from build123d import *

# Parameters (mm, degrees)
F1_DEPTH = 152.4
F2_T     = -6.35


with BuildPart() as f1:
    # F0 (on Front) → F1 (new body)
    with BuildSketch(Plane.XZ):
        with BuildLine():
            ThreePointArc((0, 9.525), (2.789808, 2.789808), (9.525, 0))
            Line((9.525, 0), (53.975, 0))
            ThreePointArc((53.975, 0), (60.710192, 2.789808), (63.5, 9.525))
            Line((63.5, 9.525), (63.5, 53.975))
            ThreePointArc((63.5, 53.975), (60.710192, 60.710192), (53.975, 63.5))
            Line((53.975, 63.5), (9.525, 63.5))
            ThreePointArc((9.525, 63.5), (2.789808, 60.710192), (0, 53.975))
            Line((0, 53.975), (0, 9.525))
        make_face()
    extrude(amount=F1_DEPTH)

    # F2
    f2_openings = [f1.faces().sort_by_distance(p)[0] for p in [
        (31.75, -152.4, 31.75),
        (31.75, 0, 31.75),
    ]]
    offset(amount=F2_T, openings=f2_openings)


solid = f1.part
Read the model definition and answer for the solid it produces. Units are mm, in the model's axes. A direction names the side the tool comes from. Give positions to 0.01 mm unless a question says otherwise; leave off trailing zeros. Write each loop counter-clockwise with the first axis right and the second up, starting at its lowest first coordinate (ties: lowest second). Pieces come first, ordered by that corner, then holes. Notation, with made-up numbers: (29.5, 24.25) - (52.5, 24.25) arc R25 ccw to (52.5, 51.25) - close; hole circle Ø2 at (16, 78). An arc over 180 degrees is marked (long way). Use CSV: the item, a comma, the result in double quotes. Start each with the question number.
Item 1: The part is cut by section B-B, the plane y = -38. Give the vertices of the cut face in (x, z) (3 decimals).
Item 2: The part is cut by section C-C, the plane z = 13.5. Give the vertices of the cut face in (x, y).
Item 3: Consider line 1 (Z direction, x = 42, y = -109.5). Determine where the line is inside the solid, lowest interval first.
Item 4: The mould has two halves that part along X. Classify faces 3 (the flat face through (57.15, -75, 31)), 4 (the cylindrical face through (60.64, -75.13, 2.72)), 5 (the cylindrical face through (2.86, -75.13, 60.78)), 6 (the flat face through (31, 0, 4)): pulls with the +X half, pulls with the -X half, needs draft (parallel to the pull), parting line crosses it, or undercut.
Item 5: The part is cut by section A-A, the plane x = 33.5. Give the vertices of the cut face in (y, z).
Item 6: Flat-ended cylindrical pins translate along their axes: P1, Ø1.5, axis at x = 8, y = -40.5, coming from the -Z side; P2, Ø12, axis at x = 17.5, z = 17.5, coming from the -Y side; P3, Ø1, axis at y = -97.5, z = 8, coming from the +X side. Find the tip coordinate at first contact, or state that the pin passes through.
Item 7: For faces 1 (the cylindrical face through (2.72, -75.13, 2.86)), 2 (the cylindrical face through (56.2, -75.13, 7.26)), determine the directions among +Z, -Z, +X, -X, +Y, -Y from which every point of the face is accessible in a straight line to the end or side of a thin tool.
Taken from the geometry:
1,outline,"(0, 9.525) arc R9.525 ccw to (9.525, 0) - (53.975, 0) arc R9.525 ccw to (63.5, 9.525) - (63.5, 53.975) arc R9.525 ccw to (53.975, 63.5) - (9.525, 63.5) arc R9.525 ccw to (0, 53.975) - close; hole (6.35, 9.525) arc R3.175 ccw to (9.525, 6.35) - (53.975, 6.35) arc R3.175 ccw to (57.15, 9.525) - (57.15, 53.975) arc R3.175 ccw to (53.975, 57.15) - (9.525, 57.15) arc R3.175 ccw to (6.35, 53.975) - close"
2,outline,"(0, -152.4) - (6.35, -152.4) - (6.35, 0) - (0, 0) - close; (57.15, -152.4) - (63.5, -152.4) - (63.5, 0) - (57.15, 0) - close"
3,line 1,"0 to 6.35, 57.15 to 63.5"
4,face 3,"undercut"
4,face 4,"pulls with the +X half"
4,face 5,"pulls with the -X half"
4,face 6,"needs draft"
5,outline,"(-152.4, 0) - (0, 0) - (0, 6.35) - (-152.4, 6.35) - close; (-152.4, 57.15) - (0, 57.15) - (0, 63.5) - (-152.4, 63.5) - close"
6,P1,"z = 0.03"
6,P2,"through"
6,P3,"x = 63.44"
7,face 1,"-Z, -X, +Y, -Y"
7,face 2,"+Y, -Y"
